Work out the finished part from the listing and answer in its coordinate system (mm). A direction names the side the tool comes from. Coordinates: 2 decimals unless noted, no trailing zeros. Order: outer loops, then holes, each group sorted by start corner. A loop starts at its lowest first (then second) coordinate and runs counter-clockwise, first axis right, second up. Notation, with made-up numbers: M 61.5,28 L 91.5,28 A23 ccw 91.5,50 Z; hole C 57,75 d1. An arc over 180 degrees is marked long. Answer in a Markdown table with one row per item. Add a question column.
Item 1: Consider line 1 (Y direction, x = 16, z = 476.5). Determine where the line is inside the solid, lowest interval first. Write a range as from..to.
Item 2: The mould has two halves that part along X. Classify faces 3 (the face through (44.45, 25, 438)), 4 (the face through (48, 26, 0)), 5 (the face through (0, 26, 438)): released by +X, released by -X, zero draft, split by the parting line, or undercut.
Item 3: The part is cut by section B-B (z = 218). Write down the section's boundary in (x, y).
Item 4: Which of the six approach directions +Z, -Z, +X, -X, +Y, -Y give full straight-line access (tool end or side, diameter ignored) to faces 1 (the face through (26, 50.8, 438)), 2 (the face through (26, 44.45, 438))?
Item 5: A flat-ended cylindrical pin translates along its axis: pin 1 Ø12 at (x, y) = (16.5, 29) entering from +Z. Find the tip coordinate at first contact, or state that the pin passes through.
Item 6: The part is cut by section A-A (y = 30.5). Write down the section's boundary in (x, z), then the cut area to 3 significant figures.
from build123d import *

# Parameters (mm, degrees)
F1_DEPTH = 889
F2_T     = 6.35


# Not quite as in the source:
# - a shell that OpenCascade refuses in one call is made with other operations: the cavity is built on its own and cut out


with BuildPart() as f1:
    # F0 (on Top) → F1 (new body)
    with BuildSketch(Plane.XY):
        with BuildLine():
            ThreePointArc((0, 6.35), (1.8598719395, 1.8598719395), (6.35, 0))
            Line((6.35, 0), (44.45, 0))
            ThreePointArc((44.45, 0), (48.9401280605, 1.8598719395), (50.8, 6.35))
            Line((50.8, 6.35), (50.8, 44.45))
            ThreePointArc((50.8, 44.45), (48.9401280605, 48.9401280605), (44.45, 50.8))
            Line((44.45, 50.8), (6.35, 50.8))
            ThreePointArc((6.35, 50.8), (1.8598719395, 48.9401280605), (0, 44.45))
            Line((0, 44.45), (0, 6.35))
        make_face()
    extrude(amount=F1_DEPTH)

    # F2: shell of thickness 6.35, made by hand


with BuildPart() as f2_core1:
    # F2_t2: copy of F1
    add(f1.part)

    # the walls: a layer under each face that stays
    f2_faces = [f2_core1.faces().sort_by_distance(p)[0] for p in [
        (0, 25.4, 444.5),
        (25.4, 0, 444.5),
        (50.8, 25.4, 444.5),
        (25.4, 50.8, 444.5),
    ]]
    thicken(f2_faces, amount=-F2_T, mode=Mode.SUBTRACT)


with BuildPart() as f1_1:
    add(f1.part)

    # what is left inside the walls is the cavity
    f2_cavity = [f2_core1.part.solids().sort_by_distance(p)[0] for p in [
        (6.4135, 25.4, 592.666667),
    ]]
    add(f2_cavity, mode=Mode.SUBTRACT)


solid = f1_1.part
Reply:
| question | item | result |
|---|---|---|
| 1 | line 1 | y = 0..6.35, 44.45..50.8 |
| 2 | face 3 | undercut |
| 2 | face 4 | zero draft |
| 2 | face 5 | released by -X |
| 3 | outline | M 0,6.35 A6.35 ccw 6.35,0 L 44.45,0 A6.35 ccw 50.8,6.35 L 50.8,44.45 A6.35 ccw 44.45,50.8 L 6.35,50.8 A6.35 ccw 0,44.45 Z; hole M 6.35,6.35 L 44.45,6.35 L 44.45,44.45 L 6.35,44.45 Z |
| 4 | face 1 | +Z, -Z, +X, -X, +Y |
| 4 | face 2 | +Z, -Z |
| 5 | pin 1 | passes through |
| 6 | outline | M 0,0 L 6.35,0 L 6.35,889 L 0,889 Z; M 44.45,0 L 50.8,0 L 50.8,889 L 44.45,889 Z |
| 6 | area | 11,300 mm2 |
